```python
from build123d import *

# Parameters (mm, degrees)
F1_DEPTH = 63.5
F2_DEPTH = 25.4
F3_DEPTH = 7.9375
F5_R     = 6.35


with BuildPart() as f1:
    # F0 (on Front) → F1 (new body, symmetric)
    with BuildSketch(Plane.XZ):
        Polygon((41.275, -9.525), (41.275, 9.525), (22.225, 9.525), (-41.275, 9.525), (-41.275, -9.525), align=None)
    extrude(amount=F1_DEPTH, both=True)

    # F0 (on Front) → F2 (join, symmetric)
    with BuildSketch(Plane.XZ):
        with BuildLine():
            Line((22.225, 9.525), (41.275, 9.525))
            Line((41.275, 9.525), (41.275, 27.0002))
            ThreePointArc((41.275, 27.0002), (45.9246798487, 38.2255201513), (57.15, 42.8752))
            Line((57.15, 42.8752), (60.325, 42.8752))
            Line((60.325, 42.8752), (60.325, 61.9252))
            Line((60.325, 61.9252), (57.15, 61.9252))
            add(Edge.make_bspline(
                [(54.6691726914, 61.8369782791), (55.5065067591, 61.8779502767), (56.3337362614, 61.9074431943), (57.15, 61.9252)],
                knots=[109.0952645489, 109.0952645489, 109.0952645489, 109.0952645489, 111.5045361635, 111.5045361635, 111.5045361635, 111.5045361635], degree=3))
            ThreePointArc((54.6691726914, 61.8369782791), (31.592236808, 50.8026445304), (22.225, 27.0002))
            Line((22.225, 27.0002), (22.225, 9.525))
        make_face()
        Polygon((60.325, 61.9252), (60.325, 42.8752), (85.8856061574, 42.8752), (85.7570526696, 61.9252), align=None)
    extrude(amount=F2_DEPTH, both=True)

    # F0 (on Front) → F3 (join, symmetric)
    with BuildSketch(Plane.XZ):
        with BuildLine():
            Line((-41.275, 9.525), (22.225, 9.525))
            Line((22.225, 9.525), (22.225, 27.0002))
            ThreePointArc((22.225, 27.0002), (31.592236808, 50.8026445304), (54.6691726914, 61.8369782791))
            add(Edge.make_bspline(
                [(-41.275, 9.525), (-41.8806763556, 34.5896402805), (16.7534885196, 59.9817076265), (54.6691726914, 61.8369782791)],
                knots=[0, 0, 0, 0, 109.0952645489, 109.0952645489, 109.0952645489, 109.0952645489], degree=3))
        make_face()
    extrude(amount=F3_DEPTH, both=True)

    # F0 (on Front) → F4 (revolve)
    with BuildSketch(Plane.XZ):
        Polygon((85.7570526696, 61.9252), (85.8856061574, 42.8752), (85.9178302317, 38.1), (111.125, 38.1), (111.125, 66.675), (85.725, 66.675), align=None)
    revolve(axis=Axis((85.8214151158, 0, 52.3875), (0.0067480609, 0, -0.9999772316)))

    # F5
    f5_edges = [f1.edges().sort_by_distance(p)[0] for p in [
        (41.275, -63.5, 0),
        (-41.275, -63.5, 0),
        (-41.275, 63.5, 0),
        (41.275, 63.5, 0),
    ]]
    fillet(f5_edges, radius=F5_R)


solid = f1.part
```
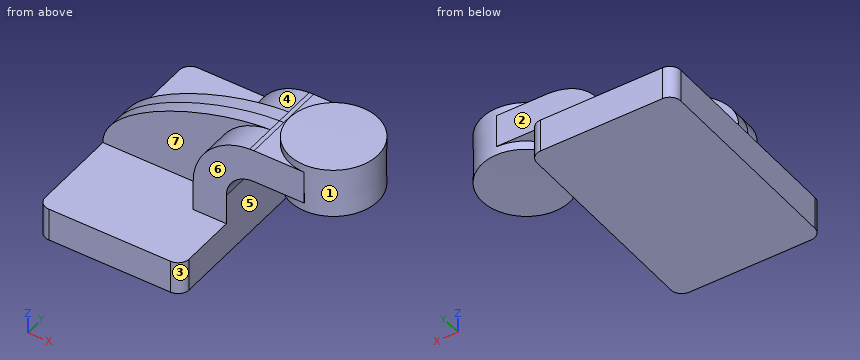
Geometry check sheet. Reference: the model listing, model coordinates, mm. Face numbers are marked on the shaded views. A direction names the side the tool comes from. Round coordinates to 2 decimals unless told otherwise and drop trailing zeros. Loops run counter-clockwise (first coordinate to the right, second up) from the corner with the lowest first, then second, coordinate; pieces in that order, holes last. Notation, with made-up numbers: (37, 49) - (88, 49) arc R11 cw to (88, 69) - close; hole circle Ø11 at (17, 46.25). An arc over 180 degrees is marked (long way). Write item = value, one per line. Start each with the question number.
1. Set-up check for the marked faces 4, 5, 6 and 7: record each of +Z, -Z, +X, -X, +Y, -Y from which the full face is reachable in a straight line by a thin tool's end or side.
2. Section check B-B on y = 31. Enter the section's corners in (x, z) (3 decimals), then the cut area to 3 significant figures.
3. Section check A-A on z = 6. Enter the section's corners in (x, y) (3 decimals), then the cut area to 3 significant figures.
4. Mould release check, pull along X, two halves, no side actions. Record for the marked faces 1, 2 and 3: released by +X, released by -X, zero draft, split by the parting line, or undercut.
5. Depth check by flat-ended pin: pin 1 (18.5 mm diameter, centred on y = 19, z = 13, fed in from +X) (3 decimals); pin 2 (14 mm diameter, centred on y = 14.5, z = 14.5, fed in from -X) (3 decimals); pin 3 (1.5 mm diameter, centred on x = 20.5, z = 42.5, fed in from +Y). Enter the tip coordinate at first touch or a pass-through.
6. Thickness scan on line 1 (Y direction, x = 17, z = 20.5); line 2 (Z direction, x = -10, y = 56.5) (3 decimals); line 3 (X direction, y = 21.5, z = -3.5) (3 decimals). Record the ranges inside material, lowest first.
Working result:
q1.face_4 = +Z, -X, +Y
q1.face_5 = -Z, +X, +Y, -Y
q1.face_6 = +Z, +X, -X, -Y
q1.face_7 = +Z, -X, -Y
q2.outline = (-41.275, -9.525) - (41.275, -9.525) - (41.275, 9.525) - (-41.275, 9.525) - close
q2.area = 1,570 mm^2
q3.outline = (-41.275, -57.15) arc R6.35 ccw to (-34.925, -63.5) - (34.925, -63.5) arc R6.35 ccw to (41.275, -57.15) - (41.275, 57.15) arc R6.35 ccw to (34.925, 63.5) - (-34.925, 63.5) arc R6.35 ccw to (-41.275, 57.15) - close
q3.area = 10,400 mm^2
q4.face_1 = undercut
q4.face_2 = zero draft
q4.face_3 = released by +X
q5.pin_1 = 41.275
q5.pin_2 = -41.275
q5.pin_3 = 7.94
q6.line_1 = -7.94 to 7.94
q6.line_2 = -9.525 to 9.525
q6.line_3 = -41.275 to 41.275
